Autodesk Fusion 360 part; units mm, degrees
sketch "Sketch1" plane through (0, 0, 0) normal (0, 0, 1) x (1, 0, 0)
  line L0 (0, 0) -> (-148, 0)
  line L1 (-148, 0) -> (-148, 57)
  line L2 (-78, 127) -> (-70, 127)
  line L3 (0, 57) -> (0, 0)
  arc A0 (0, 57) -> (-70, 127) centre (-70, 57) ccw
  arc A1 (-78, 127) -> (-148, 57) centre (-78, 57) ccw
  point P0 (0, 127)
  dimension "d1" = 148
  dimension "d2" = 127
  dimension "d3" = 70
extrude "Extrude1" add sketch "Sketch1" along normal blind 2
Read the model definition and answer for the solid it produces. Units are mm, in the model's axes. Round coordinates to 2 decimals unless told otherwise and drop trailing zeros. Write each loop counter-clockwise with the first axis right and the second up, starting at its lowest first coordinate (ties: lowest second). Pieces come first, ordered by that corner, then holes.
1. The part is cut by section C-C, the plane y = 106.5. Determine the outline of the cut face in (x, z), then the cut area to 3 significant figures.
2. The part is cut by section A-A, the plane z = 1.5. Determine the outline of the cut face in (x, y), then the cut area to 3 significant figures.
3. The part is cut by section B-B, the plane x = -125.5. Determine the outline of the cut face in (y, z), then the cut area to 3 significant figures.
4. Straight lines are drawn through the part: L1, parallel to X at y = 57.5, z = 0.65; L2, parallel to Y at x = -124.5, z = 0.6; L3, parallel to Y at x = -87.5, z = 1.25. For each, find the intervals that lie inside material, in ascending order.
Values:
1. outline: (-127.49, 0) - (-20.51, 0) - (-20.51, 2) - (-127.49, 2) - close
1. area: 214 mm2
2. outline: (-148, 0) - (0, 0) - (0, 57) arc R70 ccw to (-70, 127) - (-78, 127) arc R70 ccw to (-148, 57) - close
2. area: 16,700 mm2
3. outline: (0, 0) - (108.42, 0) - (108.42, 2) - (0, 2) - close
3. area: 217 mm2
4. L1: x = -148 to 0
4. L2: y = 0 to 109.32
4. L3: y = 0 to 126.35
